Part model, mm, in its own coordinate system. A direction names the side the tool comes from. Round coordinates to 2 decimals unless told otherwise and drop trailing zeros. Write each loop counter-clockwise with the first axis right and the second up, starting at its lowest first coordinate (ties: lowest second). Pieces come first, ordered by that corner, then holes.
from build123d import *

# Parameters (mm, degrees)
F1_DEPTH  = 16
F3_W      = 70
F3_H      = 3
F4_DEPTH  = 2
F5_W      = 50
F5_H      = 14
F6_DEPTH  = 2
F7_R      = 1
F10_DEPTH = 2
F12_DEPTH = 38.001
F14_D     = 4
F15_R     = 3
F15_R_2   = 2
F16_DEPTH = 5
F17_R     = 3


# Not quite as in the source:
# - a pattern or mirror of a feature is missing from the dataset's text; its kind, count and spacing are read off the source's solid


with BuildPart() as f1:
    # F0 (on Front) → F1 (new body)
    with BuildSketch(Plane.XZ):
        with BuildLine():
            ThreePointArc((0, -9), (-9, 0), (0, 9))
            Line((0, 9), (94, 9))
            Line((94, 9), (94, 11))
            Line((94, 11), (0, 11))
            ThreePointArc((0, 11), (-11, 0), (0, -11))
            Line((0, -11), (19, -11))
            ThreePointArc((19, -11), (21.7681124643, -11.8361612201), (23.6103896104, -14.064978646))
            ThreePointArc((23.6103896104, -14.064978646), (52.4527960943, -47.6352500016), (95.4829432523, -57.9915990802))
            ThreePointArc((95.4829432523, -57.9915990802), (101.8289994783, -58.4789828394), (107.4829432523, -61.4018055084))
            Line((107.4829432523, -61.4018055084), (109.4421656321, -61))
            ThreePointArc((109.4421656321, -61), (102.9917579834, -56.7391896111), (95.2965735981, -56))
            ThreePointArc((95.2965735981, -56), (52.955209083, -45.5949761441), (24.9861322889, -12.1467114099))
            ThreePointArc((24.9861322889, -12.1467114099), (23.1470623984, -9.8607704249), (20.3422845953, -9))
            Line((20.3422845953, -9), (0, -9))
        make_face()
    extrude(amount=F1_DEPTH)

    # F3 (on face) → F4 (join)
    with BuildSketch(Plane.XY.offset(11)):
        with Locations((59, -17.5)):
            Rectangle(F3_W, F3_H)
    extrude(amount=-F4_DEPTH)

    # F5 (on face) → F6 (join)
    with BuildSketch(Plane.XZ.offset(19)):
        with Locations((69, 4)):
            Rectangle(F5_W, F5_H)
    extrude(amount=-F6_DEPTH)

    # F7
    f7_edges = [f1.edges().sort_by_distance(p)[0] for p in [
        (59, -19, 11),
        (69, -17, 9),
    ]]
    fillet(f7_edges, radius=F7_R)

    # F8: F1 across plane


with BuildPart() as f1_1:
    add(f1.part)
    add(f1.part.mirror(Plane.XZ))

    # F9 (on face) → F10 (cut)
    with BuildSketch(Plane.XY.offset(11)):
        with BuildLine():
            Line((94, 11.964731734), (34, 11.964731734))
            ThreePointArc((34, 11.964731734), (22.9193446211, 0), (34, -11.964731734))
            Line((34, -11.964731734), (94, -11.964731734))
            Line((94, -11.964731734), (94, 11.964731734))
        make_face()
    extrude(amount=-F10_DEPTH, mode=Mode.SUBTRACT)

    # F11 (on face) → F12 (cut, through all)
    with BuildSketch(Plane.XZ.offset(19)):
        with BuildLine():
            ThreePointArc((50, 5), (47, 2), (50, -1))
            Line((50, -1), (70, -1))
            ThreePointArc((70, -1), (73, 2), (70, 5))
            Line((70, 5), (50, 5))
        make_face()
    extrude(amount=-F12_DEPTH, mode=Mode.SUBTRACT)

    # F14 (through all)
    with Locations(Plane.XZ.offset(19)):
        with Locations((80, 3)):
            Hole(F14_D / 2)

    # F15 (on face) → F16 (join)
    with BuildSketch(Plane(origin=(0, -17, 0), x_dir=(-1, 0, 0), z_dir=(0, 1, 0))):
        with Locations((-80, 3)):
            Circle(F15_R)
        with Locations((-80, 3)):
            Circle(F15_R_2, mode=Mode.SUBTRACT)
    f16 = extrude(amount=F16_DEPTH)

    # F16_copies: F16 across plane
    add(f16.mirror(Plane.ZX))

    # F17
    f17_edges = [f1_1.edges().sort_by_distance(p)[0] for p in [
        (44, -18, -3),
        (94, 18, -3),
        (94, -18, -3),
        (44, 18, -3),
    ]]
    fillet(f17_edges, radius=F17_R)


solid = f1_1.part
Q1. Tool access for faces 5 (the cylindrical face through (83, -15, 3)), 6 (the flat face through (31, 16, -25)), 7 (the cylindrical face through (47, -18, 2)): list every direction of +Z, -Z, +X, -X, +Y, -Y with a clear straight run to the whole face (end or side of a thin tool).
Q2. Saw through at C-C, the plane y = 10. Write the cut outline in (x, z).
Q3. Saw through at D-D, the plane z = 3. Give the number of separate pieces and of enclosed holes in the cut face, and give its area (4 significant figures).
Q4. Saw through at B-B, the plane y = -14.5. Write the cut outline in (x, z).
Q5. Wall check: line 1 (Z direction, x = 80, y = 17.5); line 2 (Z direction, x = 80, y = -13); line 3 (Y direction, x = 55.5, z = 5.5). Give the ranges that are in metal, low to high.
Q6. Two-plate mould, pull along Z, no slides. Class faces 1 (the cylindrical face through (23.181, -0.224, -9.884)), 2 (the flat face through (44, -18, 4)), 3 (the flat face through (10, 0, -9)), 4 (the cylindrical face through (101.743, -0.224, -58.455)): released by +Z, released by -Z, zero draft, split by the parting line, or undercut.
Q7. Saw through at A-A, the plane x = 3. Write the cut outline in (y, z), and give its area (3 significant figures).
Q8. Drop flat-ended pins along their axis: P1, Ø1.6, axis at y = 17, z = 10, coming from the -X side; P2, Ø1.5, axis at x = 68.5, y = 2.5, coming from the +Z side; P3, Ø5.5, axis at x = 10, y = -5, coming from the -Z side. Give the stop position or say it passes through.
Computed:
1. face 5: none
1. face 6: -Z, -X, +Y
1. face 7: +Y, -Y
2. outline: (0, -11) - (19, -11) arc R5 cw to (23.61, -14.06) arc R72 ccw to (95.48, -57.99) arc R16 cw to (107.48, -61.4) - (109.44, -61) arc R16 ccw to (95.3, -56) arc R70 cw to (24.99, -12.15) arc R5 ccw to (20.34, -9) - (0, -9) arc R9 cw to (0, 9) - (28.29, 9) - (28.29, 11) - (0, 11) arc R11 ccw to start
3. separate pieces: 7
3. enclosed holes: 0
3. area: 168.5 mm2
4. outline: (0, -11) - (19, -11) arc R5 cw to (23.61, -14.06) arc R72 ccw to (95.48, -57.99) arc R16 cw to (107.48, -61.4) - (109.44, -61) arc R16 ccw to (95.3, -56) arc R70 cw to (24.99, -12.15) arc R5 ccw to (20.34, -9) - (0, -9) arc R9 cw to (0, 9) - (94, 9) - (94, 11) - (0, 11) arc R11 ccw to start; circle Ø6 at (80, 3); hole circle Ø4 at (80, 3)
5. line 1: z = -3 to 1, 5 to 11
5. line 2: z = -57.5 to -55.48, 0 to 1, 5 to 6, 9 to 11
5. line 3: y = -19 to -17, 17 to 19
6. face 1: undercut
6. face 2: zero draft
6. face 3: undercut
6. face 4: released by -Z
7. outline: (-16, -11) - (16, -11) - (16, -9) - (-16, -9) - close; (-16, 9) - (16, 9) - (16, 11) - (-16, 11) - close
7. area: 128 mm2
8. P1: stops at x = 24
8. P2: stops at z = -52.57
8. P3: stops at z = -11
